Geometry check sheet. Reference: the model listing, model coordinates, mm. A direction names the side the tool comes from. Round coordinates to 2 decimals unless told otherwise and drop trailing zeros. Write each loop counter-clockwise with the first axis right and the second up, starting at its lowest first coordinate (ties: lowest second). Pieces come first, ordered by that corner, then holes.
Item 1: Scan lines: probe 1 along Z at (x, y) = (90, 6.5); probe 2 along X at (y, z) = (7.5, 0); probe 3 along X at (y, z) = (5.25, 59). Record each from-to range of solid material in increasing order.
Item 2: Cross-section at C-C (z = -26). Enter the section's corners in (x, y), then the cut area to 3 significant figures.
Item 3: Depth check by flat-ended pin: P1, Ø3, axis at y = 6, z = -39, coming from the -X side; P2, Ø3, axis at y = 7.5, z = -74, coming from the +X side; P3, Ø3, axis at y = 7, z = 60.5, coming from the +X side. Enter the tip coordinate at first touch or a pass-through.
Item 4: Draft check along X on faces 5 (the face through (93.007, 4.93, -46.242)), 6 (the face through (-66.865, 4.93, -29.944)), 7 (the face through (-68, 4.9, 30.6)). Enter one of: pulls with the +X half, pulls with the -X half, needs draft (parallel to the pull), parting line crosses it, or undercut.
Item 5: Cross-section at A-A (z = 0). Enter the section's corners in (x, y).
Item 6: Cross-section at B-B (y = 4). State how many separate pieces and enclosed holes the cut face has, then the cut area to 3 significant figures.
Item 7: Access from +Z, -Z, +X, -X, +Y, -Y to the whole of each face (thin tool, end or side, straight path). Record for faces 1 (the face through (-60.53, 4.93, -43.607)), 2 (the face through (-79.109, 5, 60)), 3 (the face through (94.109, 5, -58)), 4 (the face through (60.53, 4.93, 43.607)).
from build123d import *

# Parameters (mm, degrees)
SKETCH1_R           = 38.5
BOSS_EXTRUDE1_DEPTH = 10


with BuildPart() as part:
    # Sketch1 → Boss-Extrude1 (new body)
    with BuildSketch(Plane(origin=(0, 0, 0), x_dir=(1, 0, 0), z_dir=(0, 1, 0))):
        with BuildLine():
            Line((7.5, 49.434299833), (7.5, 99.718353376))
            ThreePointArc((7.5, 99.718353376), (6.42820323, 103.718353376), (3.5, 106.646556606))
            Line((3.5, 106.646556606), (-9.237337622, 114.000461911))
            Line((-9.237337622, 114.000461911), (-6.490381057, 118.758330249))
            ThreePointArc((-6.490381057, 118.758330249), (-24.248711306, 114), (-19.490381057, 96.241669751))
            Line((-19.490381057, 96.241669751), (-16.737337622, 101.010080854))
            Line((-16.737337622, 101.010080854), (-7.5, 95.676901492))
            Line((-7.5, 95.676901492), (-7.5, 49.434299833))
            ThreePointArc((-7.5, 49.434299833), (-25, 43.301270189), (-39.061359474, 31.212340445))
            Line((-39.061359474, 31.212340445), (-82.608627247, 56.354367216))
            ThreePointArc((-82.608627247, 56.354367216), (-86.608627247, 57.426163986), (-90.608627247, 56.354367216))
            Line((-90.608627247, 56.354367216), (-103.34596487, 49.000461911))
            Line((-103.34596487, 49.000461911), (-106.092921435, 53.758330249))
            ThreePointArc((-106.092921435, 53.758330249), (-110.851251684, 36), (-93.092921435, 31.241669751))
            Line((-93.092921435, 31.241669751), (-95.84596487, 36.010080854))
            Line((-95.84596487, 36.010080854), (-86.608627247, 41.343260217))
            Line((-86.608627247, 41.343260217), (-46.561359474, 18.221959388))
            ThreePointArc((-46.561359474, 18.221959388), (-50, 0), (-46.561359474, -18.221959388))
            Line((-46.561359474, -18.221959388), (-90.108627247, -43.36398616))
            ThreePointArc((-90.108627247, -43.36398616), (-93.036830477, -46.29218939), (-94.108627247, -50.29218939))
            Line((-94.108627247, -50.29218939), (-94.108627247, -65))
            Line((-94.108627247, -65), (-99.602540378, -65))
            ThreePointArc((-99.602540378, -65), (-86.602540378, -78), (-73.602540378, -65))
            Line((-73.602540378, -65), (-79.108627247, -65))
            Line((-79.108627247, -65), (-79.108627247, -54.333641274))
            Line((-79.108627247, -54.333641274), (-39.061359474, -31.212340445))
            ThreePointArc((-39.061359474, -31.212340445), (-25, -43.301270189), (-7.5, -49.434299833))
            Line((-7.5, -49.434299833), (-7.5, -99.718353376))
            ThreePointArc((-7.5, -99.718353376), (-6.42820323, -103.718353376), (-3.5, -106.646556606))
            Line((-3.5, -106.646556606), (9.237337622, -114.000461911))
            Line((9.237337622, -114.000461911), (6.490381057, -118.758330249))
            ThreePointArc((6.490381057, -118.758330249), (24.248711306, -114), (19.490381057, -96.241669751))
            Line((19.490381057, -96.241669751), (16.737337622, -101.010080854))
            Line((16.737337622, -101.010080854), (7.5, -95.676901492))
            Line((7.5, -95.676901492), (7.5, -49.434299833))
            ThreePointArc((7.5, -49.434299833), (25, -43.301270189), (39.061359474, -31.212340445))
            Line((39.061359474, -31.212340445), (82.608627247, -56.354367216))
            ThreePointArc((82.608627247, -56.354367216), (86.608627247, -57.426163986), (90.608627247, -56.354367216))
            Line((90.608627247, -56.354367216), (103.34596487, -49.000461911))
            Line((103.34596487, -49.000461911), (106.092921435, -53.758330249))
            ThreePointArc((106.092921435, -53.758330249), (110.851251684, -36), (93.092921435, -31.241669751))
            Line((93.092921435, -31.241669751), (95.84596487, -36.010080854))
            Line((95.84596487, -36.010080854), (86.608627247, -41.343260217))
            Line((86.608627247, -41.343260217), (46.561359474, -18.221959388))
            ThreePointArc((46.561359474, -18.221959388), (50, 0), (46.561359474, 18.221959388))
            Line((46.561359474, 18.221959388), (90.108627247, 43.36398616))
            ThreePointArc((90.108627247, 43.36398616), (93.036830477, 46.29218939), (94.108627247, 50.29218939))
            Line((94.108627247, 50.29218939), (94.108627247, 65))
            Line((94.108627247, 65), (99.602540378, 65))
            ThreePointArc((99.602540378, 65), (86.602540378, 78), (73.602540378, 65))
            Line((73.602540378, 65), (79.108627247, 65))
            Line((79.108627247, 65), (79.108627247, 54.333641274))
            Line((79.108627247, 54.333641274), (39.061359474, 31.212340445))
            ThreePointArc((39.061359474, 31.212340445), (25, 43.301270189), (7.5, 49.434299833))
        make_face()
        with Locations(Location((0, 0, 0), (0, 0, 270))):
            Circle(SKETCH1_R, mode=Mode.SUBTRACT)
        with BuildLine():
            Line((-10.490381057, 111.830127019), (2.5, 104.330127019))
            ThreePointArc((2.5, 104.330127019), (4.330127019, 97.5), (-2.5, 95.669872981))
            Line((-2.5, 95.669872981), (-15.490381057, 103.169872981))
            ThreePointArc((-15.490381057, 103.169872981), (-17.320508076, 110), (-10.490381057, 111.830127019))
        make_face(mode=Mode.SUBTRACT)
        with BuildLine():
            Line((91.602540378, 65), (91.602540378, 50))
            ThreePointArc((91.602540378, 50), (86.602540378, 45), (81.602540378, 50))
            Line((81.602540378, 50), (81.602540378, 65))
            ThreePointArc((81.602540378, 65), (86.602540378, 70), (91.602540378, 65))
        make_face(mode=Mode.SUBTRACT)
        with BuildLine():
            Line((102.092921435, -46.830127019), (89.102540378, -54.330127019))
            ThreePointArc((89.102540378, -54.330127019), (82.27241336, -52.5), (84.102540378, -45.669872981))
            Line((84.102540378, -45.669872981), (97.092921435, -38.169872981))
            ThreePointArc((97.092921435, -38.169872981), (103.923048454, -40), (102.092921435, -46.830127019))
        make_face(mode=Mode.SUBTRACT)
        with BuildLine():
            Line((10.490381057, -111.830127019), (-2.5, -104.330127019))
            ThreePointArc((-2.5, -104.330127019), (-4.330127019, -97.5), (2.5, -95.669872981))
            Line((2.5, -95.669872981), (15.490381057, -103.169872981))
            ThreePointArc((15.490381057, -103.169872981), (17.320508076, -110), (10.490381057, -111.830127019))
        make_face(mode=Mode.SUBTRACT)
        with BuildLine():
            Line((-91.602540378, -65), (-91.602540378, -50))
            ThreePointArc((-91.602540378, -50), (-86.602540378, -45), (-81.602540378, -50))
            Line((-81.602540378, -50), (-81.602540378, -65))
            ThreePointArc((-81.602540378, -65), (-86.602540378, -70), (-91.602540378, -65))
        make_face(mode=Mode.SUBTRACT)
        with BuildLine():
            Line((-102.092921435, 46.830127019), (-89.102540378, 54.330127019))
            ThreePointArc((-89.102540378, 54.330127019), (-82.27241336, 52.5), (-84.102540378, 45.669872981))
            Line((-84.102540378, 45.669872981), (-97.092921435, 38.169872981))
            ThreePointArc((-97.092921435, 38.169872981), (-103.923048454, 40), (-102.092921435, 46.830127019))
        make_face(mode=Mode.SUBTRACT)
    extrude(amount=BOSS_EXTRUDE1_DEPTH)


solid = part.part
Resolved:
1. probe 1: z = -77.55 to -68.67, -46.33 to -43.3, 39.39 to 42.26, 53.81 to 56.67
1. probe 2: x = -50 to -38.5, 38.5 to 50
1. probe 3: x = -94.11 to -91.6, -81.6 to -79.11, -7.5 to 7.5
2. outline: (-60.03, 0) - (-28.39, 0) - (-28.39, 10) - (-60.03, 10) - close; (28.39, 0) - (60.03, 0) - (60.03, 10) - (28.39, 10) - close
2. area: 633 mm2
3. P1: stops at x = -112.44
3. P2: stops at x = 97.22
3. P3: stops at x = 7.5
4. face 5: pulls with the +X half
4. face 6: undercut
4. face 7: pulls with the -X half
5. outline: (-50, 0) - (-38.5, 0) - (-38.5, 10) - (-50, 10) - close; (38.5, 0) - (50, 0) - (50, 10) - (38.5, 10) - close
6. separate pieces: 1
6. enclosed holes: 7
6. area: 9,270 mm2
7. face 1: -Z, +Y, -Y
7. face 2: +Y, -Y
7. face 3: +X, +Y, -Y
7. face 4: +Z, +Y, -Y
